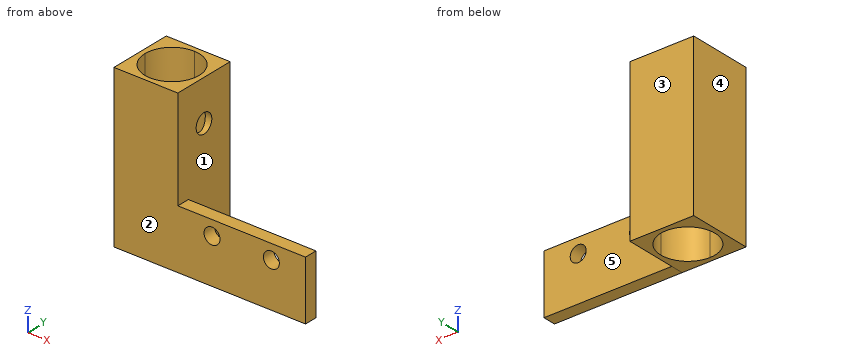
from build123d import *

# Parameters (mm, degrees)
F0_W     = 10
F0_H     = 10
F1_DEPTH = 25
F3_DEPTH = 25.001
F4_W     = 2
F4_H     = 9.304529
F5_DEPTH = 20
F7_D     = 2.5
F9_D     = 3
F9_DEPTH = 5


with BuildPart() as f1:
    # F0 (on Top) → F1 (new body)
    with BuildSketch(Plane.XY):
        with Locations((5, 5)):
            Rectangle(F0_W, F0_H)
    extrude(amount=F1_DEPTH)

    # F2 (on face) → F3 (cut, through all)
    with BuildSketch(Plane.XY.offset(25)):
        with BuildLine():
            ThreePointArc((9.25, 5), (8.005204, 8.005204), (5, 9.25))
            Line((5, 9.25), (5, 5))
            Line((5, 5), (9.25, 5))
        make_face()
        with BuildLine():
            Line((5, 5), (5, 9.25))
            ThreePointArc((5, 9.25), (1.994796, 8.005204), (0.75, 5))
            Line((0.75, 5), (5, 5))
        make_face()
        with BuildLine():
            Line((9.25, 5), (5, 5))
            Line((5, 5), (5, 0.75))
            ThreePointArc((5, 0.75), (8.005204, 1.994796), (9.25, 5))
        make_face()
        with BuildLine():
            Line((5, 0.75), (5, 5))
            Line((5, 5), (0.75, 5))
            ThreePointArc((0.75, 5), (1.994796, 1.994796), (5, 0.75))
        make_face()
    extrude(amount=-F3_DEPTH, mode=Mode.SUBTRACT)

    # F4 (on face) → F5 (join)
    with BuildSketch(Plane.YZ.offset(10)):
        with Locations((1, 4.652264)):
            Rectangle(F4_W, F4_H)
    extrude(amount=F5_DEPTH)

    # F7 (through all)
    with Locations(Plane(origin=(0, 2, 0), x_dir=(-1, 0, 0), z_dir=(0, 1, 0))):
        with Locations((-15.35, 7), (-24.65, 7)):
            Hole(F7_D / 2)

    # F9
    with Locations(Plane.YZ.offset(10)):
        with Locations((5, 18.594904)):
            Hole(F9_D / 2, depth=F9_DEPTH)


solid = f1.part
For this review, take the finished solid that the model builds, in its own axes (mm). Face numbers are marked on the shaded views. A direction names the side the tool comes from. Round coordinates to 2 decimals unless told otherwise and drop trailing zeros. Write each loop counter-clockwise with the first axis right and the second up, starting at its lowest first coordinate (ties: lowest second). Pieces come first, ordered by that corner, then holes. Notation, with made-up numbers: M -40,84 L 3,84 A17 cw 3,93 Z; hole C -35,55.25 d2. An arc over 180 degrees is marked long. Write item = value, one per line. Start each with the question number.
(1) We need section B-B (x = 15.35). Give the boundary of the cut face in (y, z).
(2) For line 1 along Z through (x, y) = (9.45, 5); line 2 along Y through (x, z) = (9.5, 18.5); line 3 along Y through (x, z) = (22.25, 6.25), list the stretches that pass through material, from the lowest coordinate up.
(3) We need section C-C (z = 2.25). Give the boundary of the cut face in (x, y).
(4) We need section A-A (z = 7). Give the boundary of the cut face in (x, y), then the cut area to 3 significant figures.
(5) Clearance check with flat-ended pins moving along their axes: pin 1 Ø4 at (x, y) = (4.5, 7) entering from -Z; pin 2 Ø4 at (x, z) = (25, 7) entering from +Y; pin 3 Ø5 at (y, z) = (5, 18.59) entering from +X; pin 4 Ø2 at (x, y) = (16.5, 1) entering from +Z. State where each tip first meets the part, or that it passes through.
(6) For the marked faces 4 and 5, list the 3-axis set-ups (+Z, -Z, +X, -X, +Y, -Y) from which the entire face can be reached by the end or side of a thin tool; tool diameter is ignored.
(7) The part is to be moulded in two halves that separate along Y. For the marked faces 1, 2 and 3, say which applies: +Y half, -Y half, draft (parallel to the pull), parting line (faces both ways), or undercut.
(8) We need section D-D (y = 7.75). Give the boundary of the cut face in (x, z), then the cut area to 3 significant figures.
Results found:
q1.outline = M 0,0 L 2,0 L 2,5.75 L 0,5.75 Z; M 0,8.25 L 2,8.25 L 2,9.3 L 0,9.3 Z
q2.line_1 = 0 to 17.09, 20.09 to 25
q2.line_2 = 0 to 3.5, 6.5 to 10
q2.line_3 = 0 to 2
q3.outline = M 0,0 L 30,0 L 30,2 L 10,2 L 10,10 L 0,10 Z; hole M 0.75,5 A4.25 ccw 5,0.75 A4.25 ccw 9.25,5 A4.25 ccw 5,9.25 A4.25 ccw Z
q4.outline = M 0,0 L 14.1,0 L 14.1,2 L 10,2 L 10,10 L 0,10 Z; M 16.6,0 L 23.4,0 L 23.4,2 L 16.6,2 Z; M 25.9,0 L 30,0 L 30,2 L 25.9,2 Z; hole M 0.75,5 A4.25 ccw 5,0.75 A4.25 ccw 9.25,5 A4.25 ccw 5,9.25 A4.25 ccw Z
q4.area = 73.3 mm²
q5.pin_1 = through
q5.pin_2 = 2
q5.pin_3 = 10
q5.pin_4 = 9.3
q6.face_4 = +Z, -Z, -X, +Y, -Y
q6.face_5 = +Z, -Z, +X, +Y
q7.face_1 = draft
q7.face_2 = -Y half
q7.face_3 = +Y half
q8.outline = M 0,0 L 1.76,0 L 1.76,25 L 0,25 Z; M 8.24,0 L 10,0 L 10,25 L 8.24,25 Z
q8.area = 88.0 mm²
